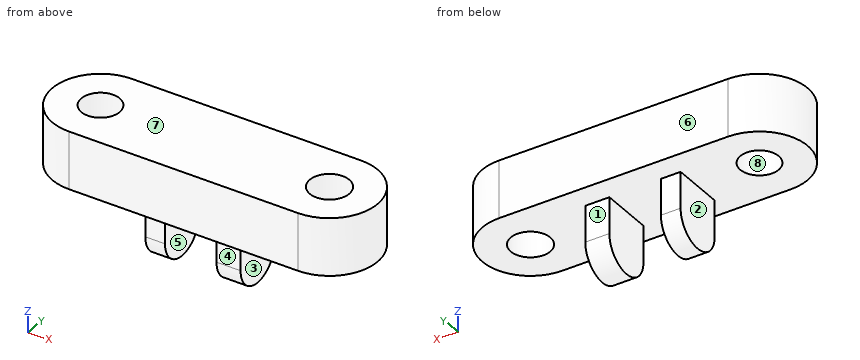
from build123d import *

# Parameters (mm, degrees)
F0_R     = 8.4622870675
F0_R_2   = 8.7058522528
F1_DEPTH = 25.4
F2_W     = 8.6757829413
F2_H     = 23.0149254203
F2_W_2   = 10.6037370861
F3_DEPTH = 16.002
F4_W     = 8.6757829413
F4_H     = 11.5074627101
F6_W     = 10.6037370861
F6_H     = 11.5074627101


with BuildPart() as f1:
    # F0 (on Top) → F1 (new body)
    with BuildSketch(Plane.XY):
        with BuildLine():
            Line((58.2000501454, 33.3776660264), (-42.5354391336, 33.3776660264))
            ThreePointArc((-42.5354391336, 33.3776660264), (-63.7429091148, 12.1701960452), (-42.5354391336, -9.037273936))
            Line((-42.5354391336, -9.037273936), (58.2000501454, -9.037273936))
            ThreePointArc((58.2000501454, -9.037273936), (79.4075201266, 12.1701960452), (58.2000501454, 33.3776660264))
        make_face()
        with Locations((-42.5354391336, 12.1701960452)):
            Circle(F0_R, mode=Mode.SUBTRACT)
        with Locations((58.2000501454, 12.1701960452)):
            Circle(F0_R_2, mode=Mode.SUBTRACT)
    extrude(amount=F1_DEPTH)

    # F2 (on Top) → F3 (join)
    with BuildSketch(Plane.XY):
        with Locations((-10.56643622, 11.5074627101)):
            Rectangle(F2_W, F2_H)
        with Locations((21.726757288, 11.5074627101)):
            Rectangle(F2_W_2, F2_H)
    extrude(amount=-F3_DEPTH)

    # F4 (on face) → F5 (revolve)
    with BuildSketch(Plane(origin=(0, 0, -16.002), x_dir=(1, 0, 0), z_dir=(0, 0, -1))):
        with Locations((-10.56643622, -5.7537313551)):
            Rectangle(F4_W, F4_H)
    revolve(axis=Axis((-10.56643622, 11.5074627101, -16.002), (1, 0, 0)))

    # F6 (on face) → F7 (revolve)
    with BuildSketch(Plane(origin=(0, 0, -16.002), x_dir=(1, 0, 0), z_dir=(0, 0, -1))):
        with Locations((21.726757288, -5.7537313551)):
            Rectangle(F6_W, F6_H)
    revolve(axis=Axis((21.726757288, 11.5074627101, -16.002), (1, 0, 0)))


solid = f1.part
Can you work these out from the model? Positions are in its coordinate system, mm. Face numbers are marked on the shaded views. A direction names the side the tool comes from. Round coordinates to 2 decimals unless told otherwise and drop trailing zeros. Write each loop counter-clockwise with the first axis right and the second up, starting at its lowest first coordinate (ties: lowest second). Pieces come first, ordered by that corner, then holes. Notation, with made-up numbers: (-31.5, -2) -> (4.5, -2) arc R33 ccw to (4.5, 32) -> close; hole circle Ø1 at (-27.75, 40). An arc over 180 degrees is marked (long way). Use one line per item in the form item = value. Start each with the question number.
Q1. Imagine slicing it at B-B (y = 8). Please give me the cut outline in (x, z), then the cut area to 3 significant figures.
Q2. If I drill on probe 1 along X at (y, z) = (11.5, 10); probe 2 along X at (y, z) = (11, -16); probe 3 along Y at (x, z) = (58.5, 9), over which ranges is the centre line in solid material (lowest first)? Write a range as [from, to].
Q3. Imagine slicing it at D-D (x = 53). Please give me the cut outline in (y, z), then the cut area to 3 significant figures.
Q4. Which directions (+Z, -Z, +X, -X, +Y, -Y) give clear straight access to the entire face, cutting with the end or side of a thin tool? Please do the marked faces 1, 2, 3, 4 and 5.
Q5. Imagine slicing it at A-A (z = -10). Please give me the cut outline in (x, y), then the cut area to 3 significant figures.
Q6. We'd pull the mould along Y, two halves only. Please class the marked faces 6, 7 and 8: +Y half, -Y half, draft (parallel to the pull), parting line (faces both ways), or undercut.
Q7. I'm going to push flat-ended pins straight in: P1, Ø10, axis at y = 4, z = 18, coming from the +X side; P2, Ø8, axis at y = 15.5, z = -12.5, coming from the +X side; P3, Ø8, axis at x = -3.5, z = -22, coming from the +Y side. Where does each tip first touch, or does it pass through?
Worked out:
q1.outline = (-63.33, 0) -> (-49.9, 0) -> (-49.9, 25.4) -> (-63.33, 25.4) -> close; (-35.17, 0) -> (-14.9, 0) -> (-14.9, -26.96) -> (-6.23, -26.96) -> (-6.23, 0) -> (16.42, 0) -> (16.42, -26.96) -> (27.03, -26.96) -> (27.03, 0) -> (50.56, 0) -> (50.56, 25.4) -> (-35.17, 25.4) -> close; (65.84, 0) -> (78.99, 0) -> (78.99, 25.4) -> (65.84, 25.4) -> close
q1.area = 3,370 mm^2
q2.probe_1 = [-63.73, -50.97], [-34.1, 49.52], [66.88, 79.4]
q2.probe_2 = [-14.9, -6.23], [16.42, 27.03]
q2.probe_3 = [-9.04, 3.47], [20.87, 33.38]
q3.outline = (-9.04, 0) -> (5.19, 0) -> (5.19, 25.4) -> (-9.04, 25.4) -> close; (19.15, 0) -> (33.38, 0) -> (33.38, 25.4) -> (19.15, 25.4) -> close
q3.area = 723 mm^2
q4.face_1 = -Z, +X, -X, +Y
q4.face_2 = -Z, -X, +Y, -Y
q4.face_3 = -Z, +X, +Y, -Y
q4.face_4 = -Z, +X, -X, -Y
q4.face_5 = -Z, +Y, -Y
q5.outline = (-14.9, 0) -> (-6.23, 0) -> (-6.23, 23.01) -> (-14.9, 23.01) -> close; (16.42, 0) -> (27.03, 0) -> (27.03, 23.01) -> (16.42, 23.01) -> close
q5.area = 444 mm^2
q6.face_6 = +Y half
q6.face_7 = draft
q6.face_8 = undercut
q7.P1 = 79.17
q7.P2 = 27.03
q7.P3 = 22.6
